Verification items for the finished model (mm, model axes). A direction names the side the tool comes from. Give positions to 0.01 mm unless a question says otherwise; leave off trailing zeros. Write each loop counter-clockwise with the first axis right and the second up, starting at its lowest first coordinate (ties: lowest second). Pieces come first, ordered by that corner, then holes. Notation, with made-up numbers: (3.25, -4) -> (27.25, -4) arc R21 ccw to (27.25, 1) -> close; hole circle Ø5 at (36, 52). An arc over 180 degrees is marked (long way). Answer as CSV lines item,"result".
```python
from build123d import *

# Parameters (mm, degrees)
SKETCH_1_W          = 135
SKETCH_1_H          = 40
EXTRUDE_310_DEPTH   = 68
SKETCH_2_W          = 39
SKETCH_2_H          = 15
CUT_EXTRUDE_1_DEPTH = 66
SKETCH_4_W          = 53
SKETCH_4_H          = 9.428155193
CUT_EXTRUDE_2_DEPTH = 66
SKETCH_6_W          = 53
SKETCH_6_H          = 10.153175229
CUT_EXTRUDE_3_DEPTH = 66
SKETCH_7_W          = 30.334064535
SKETCH_7_H          = 3
SKETCH_7_W_2        = 33.750062794
SKETCH_7_W_3        = 31.017264187
CUT_EXTRUDE_4_DEPTH = 66


with BuildPart() as part:
    # Эскиз1 → Extrude 310 (new body)
    with BuildSketch(Plane(origin=(0, 0, 0), x_dir=(1, 0, 0), z_dir=(0, 1, 0))):
        with Locations((67.5, 20)):
            Rectangle(SKETCH_1_W, SKETCH_1_H)
    extrude(amount=EXTRUDE_310_DEPTH)

    # Эскиз2 → Вырез-Вытянуть1 (cut)
    with BuildSketch(Plane.XZ):
        with Locations((21.5, -10.5)):
            Rectangle(SKETCH_2_W, SKETCH_2_H)
        with Locations((67.5, -10.5)):
            Rectangle(SKETCH_2_W, SKETCH_2_H)
        with Locations((113.5, -10.5)):
            Rectangle(SKETCH_2_W, SKETCH_2_H)
        with Locations((67.5, -28.5)):
            Rectangle(SKETCH_2_W, SKETCH_2_H)
        with Locations((113.5, -28.5)):
            Rectangle(SKETCH_2_W, SKETCH_2_H)
        with Locations((21.5, -28.5)):
            Rectangle(SKETCH_2_W, SKETCH_2_H)
    extrude(amount=-CUT_EXTRUDE_1_DEPTH, mode=Mode.SUBTRACT)

    # Эскиз4 → Вырез-Вытянуть2 (cut)
    with BuildSketch(Plane.XZ):
        with Locations((67.5, -10.503524842)):
            Rectangle(SKETCH_4_W, SKETCH_4_H)
    extrude(amount=-CUT_EXTRUDE_2_DEPTH, mode=Mode.SUBTRACT)

    # Эскиз6 → Вырез-Вытянуть3 (cut)
    with BuildSketch(Plane.XZ):
        with Locations((67.5, -28.288326327)):
            Rectangle(SKETCH_6_W, SKETCH_6_H)
    extrude(amount=-CUT_EXTRUDE_3_DEPTH, mode=Mode.SUBTRACT)

    # Эскиз7 → Вырез-Вытянуть4 (cut)
    with BuildSketch(Plane.XZ):
        with Locations((22.818742778, -19.5)):
            Rectangle(SKETCH_7_W, SKETCH_7_H)
        with Locations((67.158400174, -19.5)):
            Rectangle(SKETCH_7_W_2, SKETCH_7_H)
        with Locations((112.112937257, -19.5)):
            Rectangle(SKETCH_7_W_3, SKETCH_7_H)
    extrude(amount=-CUT_EXTRUDE_4_DEPTH, mode=Mode.SUBTRACT)


solid = part.part
```
1) Section check A-A (y = 57). State how many separate pieces and enclosed holes the cut face has, and give its area (3 significant figures).
Reported:
separate pieces,"3"
enclosed holes,"1"
area,"1,330 mm²"
2) Section check C-C (z = -25). Record the boundary of the cut face in (x, y).
Reported:
outline,"(0, 0) -> (2, 0) -> (2, 66) -> (133, 66) -> (133, 0) -> (135, 0) -> (135, 68) -> (0, 68) -> close"
3) Section check D-D (x = 88.5). Record the boundary of the cut face in (y, z).
Reported:
outline,"(0, -40) -> (68, -40) -> (68, 0) -> (0, 0) -> (0, -5.79) -> (66, -5.79) -> (66, -15.22) -> (0, -15.22) -> (0, -23.21) -> (66, -23.21) -> (66, -33.36) -> (0, -33.36) -> close"
4) Tool access check on faces 3 (the flat face through (67, 33, -36)), 4 (the flat face through (0, 34, -20)). Record the directions out of +Z, -Z, +X, -X, +Y, -Y that give a thin tool (end or side, any length) a straight path to the whole face; none if there is none.
Reported:
face 3,"-Y"
face 4,"+Z, -Z, -X, +Y, -Y"
5) Section check B-B (x = 107). Record the boundary of the cut face in (y, z), and give its area (3 significant figures).
Reported:
outline,"(0, -40) -> (68, -40) -> (68, 0) -> (0, 0) -> (0, -3) -> (66, -3) -> (66, -36) -> (0, -36) -> close"
area,"542 mm²"
6) Scan lines: line 1 along Z through (x, y) = (40.5, 47); line 2 along X through (y, z) = (64, -18.5); line 3 along X through (y, z) = (36, -23). Record each from-to range of solid material in increasing order.
Reported:
line 1,"-40 to -36, -21 to -18, -3 to 0"
line 2,"0 to 7.65, 37.99 to 50.28, 84.03 to 96.6, 127.62 to 135"
line 3,"0 to 2, 41 to 48, 87 to 94, 133 to 135"
7) Depth check by flat-ended pin: pin 1 (6 mm diameter, centred on x = 61.5, z = -15, fed in from -Y). Enter the tip coordinate at first touch or a pass-through.
Reported:
pin 1,"y = 66"
8) Draft check along Z on faces 1 (the flat face through (44, 0, -19)), 2 (the flat face through (67, 33, -3)). Enter one of: +Z half, -Z half, draft (parallel to the pull), parting line (faces both ways), or undercut.
Reported:
face 1,"draft"
face 2,"undercut"
